from build123d import *

# Parameters (mm, degrees)
F0_R     = 25
F1_DEPTH = 40
F2_R     = 15
F3_DEPTH = 20
F5_DEPTH = 12
F6_W     = 16
F6_H     = 16
F7_DEPTH = 12
F8_W     = 16
F8_H     = 16
F9_DEPTH = 12


with BuildPart() as f1:
    # F0 (on Top) → F1 (new body)
    with BuildSketch(Plane.XY):
        Circle(F0_R)
    extrude(amount=F1_DEPTH)

    # F2 (on face) → F3 (cut)
    with BuildSketch(Plane.XY.offset(40)):
        Circle(F2_R)
    extrude(amount=-F3_DEPTH, mode=Mode.SUBTRACT)

    # F4 (on face) → F5 (join)
    with BuildSketch(Plane(origin=(0, 0, 0), x_dir=(1, 0, 0), z_dir=(0, 0, -1))):
        with BuildLine():
            Line((50.0656880438, 20), (15, 20))
            ThreePointArc((15, 20), (22.360679775, 11.1803398875), (25, 0))
            ThreePointArc((25, 0), (22.360679775, -11.1803398875), (15, -20))
            Line((15, -20), (50.0656880438, -20))
            Line((50.0656880438, -20), (50.0656880438, 20))
        make_face()
        with BuildLine():
            Line((-15, 20), (-49.9343119562, 20))
            Line((-49.9343119562, 20), (-49.9343119562, -20))
            Line((-49.9343119562, -20), (-15, -20))
            ThreePointArc((-15, -20), (-25, 0), (-15, 20))
        make_face()
        with BuildLine():
            Line((15, 20), (-15, 20))
            ThreePointArc((-15, 20), (-25, 0), (-15, -20))
            Line((-15, -20), (15, -20))
            ThreePointArc((15, -20), (22.360679775, -11.1803398875), (25, 0))
            ThreePointArc((25, 0), (22.360679775, 11.1803398875), (15, 20))
        make_face()
    extrude(amount=-F5_DEPTH)

    # F6 (on face) → F7 (cut)
    with BuildSketch(Plane.XY.offset(12)):
        with Locations((-41.9343119562, 0)):
            Rectangle(F6_W, F6_H)
    extrude(amount=-F7_DEPTH, mode=Mode.SUBTRACT)

    # F8 (on face) → F9 (cut)
    with BuildSketch(Plane.XY.offset(12)):
        with Locations((42.0656880438, 0)):
            Rectangle(F8_W, F8_H)
    extrude(amount=-F9_DEPTH, mode=Mode.SUBTRACT)


solid = f1.part
Input: part model. Units: mm. Frame: model coordinates. A direction names the side the tool comes from. Coordinates: 2 decimals unless noted, no trailing zeros. Loops run counter-clockwise (first coordinate to the right, second up) from the corner with the lowest first, then second, coordinate; pieces in that order, holes last.
(1) Set-up query: faces 1 (the face through (42, -8, 6)), 2 (the face through (-33, 20, 6)), 3 (the face through (32, 20, 6)), 4 (the face through (-42, 8, 6)), 5 (the face through (33, -20, 6)). Return all of +Z, -Z, +X, -X, +Y, -Y with unobstructed straight access to the full face (end or side cutting, diameter ignored); none if empty.
(2) First-contact query: pin 1 Ø6 at (y, z) = (0, 4.5) entering from +X; pin 2 Ø9.5 at (x, z) = (40.5, 6) entering from -Y; pin 3 Ø13 at (x, z) = (45.5, 5) entering from +Y; pin 4 Ø24 at (x, y) = (1, 6) entering from +Z. Flat tips, straight axial feed; report the tip coordinate or a pass-through.
(3) Material intervals for probe 1 along Y at (x, z) = (0, 31); probe 2 along Z at (x, y) = (31, -16); probe 3 along X at (y, z) = (-4, 2.5), sorted ascending.
(4) Section D-D on z = 19. Return the cut outline in (x, y), then the cut area to 3 significant figures.
(5) Pull-direction query (Y, two-part tool) for faces 6 (the face through (-32, -20, 6)), 7 (the face through (50.066, 14, 6)), 8 (the face through (-14.985, 0.66, 30.14)); classes: released by +Y, released by -Y, zero draft, split by the parting line, or undercut.
(6) Section C-C on z = 28. Return the cut outline in (x, y).
(7) Section B-B on x = 0. Return the cut outline in (y, z).
(8) Section A-A on y = 0. Return the cut outline in (x, z), then the cut area to 3 significant figures.
Data:
1. face 1: +Z, -Z, +X
1. face 2: +Z, -Z, -X, +Y
1. face 3: +Z, -Z, +X, +Y
1. face 4: +Z, -Z, -X
1. face 5: +Z, -Z, +X, -Y
2. pin 1: stops at x = 34.07
2. pin 2: stops at y = -20
2. pin 3: stops at y = 20
2. pin 4: stops at z = 40
3. probe 1: y = -25 to -15, 15 to 25
3. probe 2: z = 0 to 12
3. probe 3: x = -33.93 to 34.07
4. outline: circle Ø50 at (0, 0)
4. area: 1,960 mm2
5. face 6: released by -Y
5. face 7: zero draft
5. face 8: undercut
6. outline: circle Ø50 at (0, 0); hole circle Ø30 at (0, 0)
7. outline: (-25, 0) - (25, 0) - (25, 40) - (15, 40) - (15, 20) - (-15, 20) - (-15, 40) - (-25, 40) - close
8. outline: (-33.93, 0) - (34.07, 0) - (34.07, 12) - (25, 12) - (25, 40) - (15, 40) - (15, 20) - (-15, 20) - (-15, 40) - (-25, 40) - (-25, 12) - (-33.93, 12) - close
8. area: 1,620 mm2
